Build history of the part. All positions in model axes, mm. A direction names the side the tool comes from. Round coordinates to 2 decimals unless told otherwise and drop trailing zeros. Loops run counter-clockwise (first coordinate to the right, second up) from the corner with the lowest first, then second, coordinate; pieces in that order, holes last. Notation, with made-up numbers: (70.25, 31.5) -> (111.25, 31.5) arc R28 cw to (111.25, 67.5) -> close; hole circle Ø2 at (86, 16). An arc over 180 degrees is marked (long way). Put each result on its own line as item: value. Start each with the question number.
Item 1: Pull direction X, two halves, no side cores. Call faces 4 (the cylindrical face through (36.99, -2.85, 9.86)), 5 (the flat face through (10, -20, -10)), 6 (the cylindrical face through (2.17, -9.76, 9.86)): +X half, -X half, draft (parallel to the pull), parting line (faces both ways), or undercut.
Item 2: Flat gauge pins, fed straight in: pin 1 Ø3 at (x, z) = (23.5, 5.5) entering from +Y; pin 2 Ø10 at (x, y) = (24.5, -7) entering from -Z; pin 3 Ø1 at (y, z) = (6, -1.5) entering from +X; pin 4 Ø16 at (x, z) = (4.5, -12.5) entering from +Y. Where does each tip first touch, or does it go through?
Item 3: Cut at D-D, the plane x = 26. List the corners of the cut face in (y, z), plus the area to 3 significant figures.
Item 4: Drill centre lines: probe 1 along Y at (x, z) = (0, 4); probe 2 along Y at (x, z) = (-16, -8); probe 3 along Z at (x, y) = (22.5, -0.5). Where is each one in solid material? Low to high. Write a range as [from, to].
Item 5: Cut at C-C, the plane z = 7. List the corners of the cut face in (x, y), plus the area to 3 significant figures.
Item 6: Cut at B-B, the plane y = -2.5. List the corners of the cut face in (x, z).
Item 7: Cut at A-A, the plane x = 0. List the corners of the cut face in (y, z), plus the area to 3 significant figures.
Item 8: Tool access for faces 1 (the flat face through (25, 0, 10)), 2 (the flat face through (10, -25, -20)), 3 (the flat face through (10, -4, 0)): list every direction of +Z, -Z, +X, -X, +Y, -Y with a clear straight run to the whole face (end or side of a thin tool).
```python
from build123d import *

# Parameters (mm, degrees)
BOSS_EXTRUDE4_DEPTH = 20
SKETCH6_W           = 60
SKETCH6_H           = 10
BOSS_EXTRUDE6_DEPTH = 40
SKETCH7_R           = 10
CUT_EXTRUDE2_DEPTH  = 40


with BuildPart() as part:
    # Sketch1 → Boss-Extrude4 (new body)
    with BuildSketch(Plane.XY):
        with BuildLine():
            Line((20, 0), (30, 0))
            ThreePointArc((30, 0), (37.071067812, -2.928932188), (40, -10))
            Line((40, -10), (40, -20))
            Line((40, -20), (-20, -20))
            Line((-20, -20), (-20, 0))
            ThreePointArc((-20, 0), (0, 20), (20, 0))
        make_face()
    extrude(amount=BOSS_EXTRUDE4_DEPTH)

    # Sketch6 → Boss-Extrude6 (add)
    with BuildSketch(Plane.XY.offset(20)):
        with Locations((10, -25)):
            Rectangle(SKETCH6_W, SKETCH6_H)
    extrude(amount=-BOSS_EXTRUDE6_DEPTH)

    # Sketch7 → Cut-Extrude2 (cut)
    with BuildSketch(Plane(origin=(0, 0, 0), x_dir=(-1, 0, 0), z_dir=(0, 0, -1))):
        Circle(SKETCH7_R)
    extrude(amount=-CUT_EXTRUDE2_DEPTH, mode=Mode.SUBTRACT)


solid = part.part
```
Reply:
1. face 4: +X half
1. face 5: draft
1. face 6: undercut
2. pin 1: stops at y = 0
2. pin 2: stops at z = 0
2. pin 3: passes through
2. pin 4: stops at y = -20
3. outline: (-30, -20) -> (-20, -20) -> (-20, 0) -> (0, 0) -> (0, 20) -> (-30, 20) -> close
3. area: 800 mm^2
4. probe 1: y = [-30, -10], [10, 20]
4. probe 2: y = [-30, -20]
4. probe 3: z = [0, 20]
5. outline: (-20, -30) -> (40, -30) -> (40, -10) arc R10 ccw to (30, 0) -> (20, 0) arc R20 ccw to (-20, 0) -> close; hole circle Ø20 at (0, 0)
5. area: 2,090 mm^2
6. outline: (-20, 0) -> (-9.68, 0) -> (-9.68, 20) -> (-20, 20) -> close; (9.68, 0) -> (36.61, 0) -> (36.61, 20) -> (9.68, 20) -> close
7. outline: (-30, -20) -> (-20, -20) -> (-20, 0) -> (-10, 0) -> (-10, 20) -> (-30, 20) -> close; (10, 0) -> (20, 0) -> (20, 20) -> (10, 20) -> close
7. area: 800 mm^2
8. face 1: +Z, -Z, +X, +Y
8. face 2: -Z, +X, -X, +Y, -Y
8. face 3: -Z, +X, -X, +Y
